The listing builds one solid part. Answer for the finished solid, in the listing's coordinates (mm). Face numbers are marked on the shaded views. A direction names the side the tool comes from. Coordinates: 2 decimals unless noted, no trailing zeros. Order: outer loops, then holes, each group sorted by start corner. A loop starts at its lowest first (then second) coordinate and runs counter-clockwise, first axis right, second up. Notation, with made-up numbers: (79, -40) -> (118, -40) arc R21 cw to (118, -23) -> close; hole circle Ø5 at (-6.5, 49). An arc over 180 degrees is marked (long way). One line per question, with ' | ' between items.
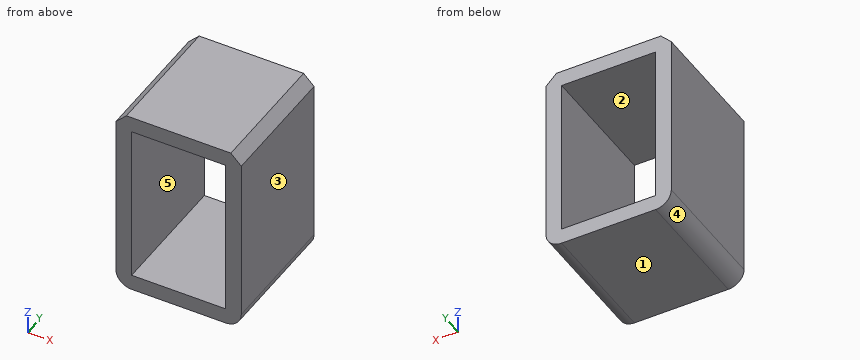
from build123d import *

# Parameters (mm, degrees)
SKETCH1_W           = 24
SKETCH1_H           = 36.6
BOSS_EXTRUDE1_DEPTH = 24.4
SKETCH2_W           = 18
SKETCH2_H           = 30.6
CUT_EXTRUDE1_DEPTH  = 24.4
FILLET2_R           = 3
CHAMFER1_SIZE       = 2


with BuildPart() as part:
    # Sketch1 → Boss-Extrude1 (new body)
    with BuildSketch(Plane(origin=(0, 0, 0), x_dir=(1, 0, 0), z_dir=(0, 1, 0))):
        with Locations((12, 18.3)):
            Rectangle(SKETCH1_W, SKETCH1_H)
    extrude(amount=BOSS_EXTRUDE1_DEPTH)

    # Sketch2 → Cut-Extrude1 (cut)
    with BuildSketch(Plane(origin=(0, 24.4, 0), x_dir=(1, 0, 0), z_dir=(0, 1, 0))):
        with Locations((12, 18.3)):
            Rectangle(SKETCH2_W, SKETCH2_H)
    extrude(amount=-CUT_EXTRUDE1_DEPTH, mode=Mode.SUBTRACT)

    # Fillet2
    fillet2_edges = [part.edges().sort_by_distance(p)[0] for p in [
        (0, 12.2, -36.6),
        (24, 12.2, -36.6),
    ]]
    fillet(fillet2_edges, radius=FILLET2_R)

    # Chamfer1
    chamfer1_edges = [part.edges().sort_by_distance(p)[0] for p in [
        (24, 12.2, 0),
        (0, 12.2, 0),
    ]]
    chamfer(chamfer1_edges, length=CHAMFER1_SIZE)


solid = part.part
Item 1: For the marked faces 1 and 2, determine the directions among +Z, -Z, +X, -X, +Y, -Y from which every point of the face is accessible in a straight line to the end or side of a thin tool.
Computed values:
face 1: -Z, +X, -X, +Y, -Y | face 2: +Y, -Y
Item 2: Find the intervals of material crossed by L1, parallel to Z at x = 3.5, y = 23.75; L2, parallel to X at y = 19, z = -31; L3, parallel to X at y = 12.75, z = -34.5, in increasing order.
Computed values:
L1: z = -36.6 to -33.6, -3 to 0 | L2: x = 0 to 3, 21 to 24 | L3: x = 0.14 to 23.86
Item 3: Section B-B, the plane x = 7 is taken. Give the vertices of the cut face in (y, z).
Computed values:
outline: (0, -36.6) -> (24.4, -36.6) -> (24.4, -33.6) -> (0, -33.6) -> close; (0, -3) -> (24.4, -3) -> (24.4, 0) -> (0, 0) -> close
Item 4: Section A-A, the plane z = -25.5 is taken. Give the vertices of the cut face in (x, y).
Computed values:
outline: (0, 0) -> (3, 0) -> (3, 24.4) -> (0, 24.4) -> close; (21, 0) -> (24, 0) -> (24, 24.4) -> (21, 24.4) -> close
Item 5: Section C-C, the plane y = 11.25 is taken. Give the vertices of the cut face in (x, z).
Computed values:
outline: (0, -33.6) arc R3 ccw to (3, -36.6) -> (21, -36.6) arc R3 ccw to (24, -33.6) -> (24, -2) -> (22, 0) -> (2, 0) -> (0, -2) -> close; hole (3, -33.6) -> (21, -33.6) -> (21, -3) -> (3, -3) -> close
Item 6: Determine the mould class of the marked faces 3, 4 and 5 for opening direction Z: pulls with the +Z half, pulls with the -Z half, needs draft (parallel to the pull), parting line crosses it, or undercut.
Computed values:
face 3: needs draft | face 4: pulls with the -Z half | face 5: undercut
